Geometry check sheet. Reference: the model listing, model coordinates, mm. A direction names the side the tool comes from. Coordinates: 2 decimals unless noted, no trailing zeros. Order: outer loops, then holes, each group sorted by start corner. A loop starts at its lowest first (then second) coordinate and runs counter-clockwise, first axis right, second up. Notation, with made-up numbers: (-32.75, 3) - (10.25, 3) arc R23 cw to (10.25, 40) - close; hole circle Ø8 at (76.25, 23). An arc over 180 degrees is marked (long way). Put each result on its own line as item: value.
from build123d import *

# Parameters (mm, degrees)
SKETCH2_W           = 18.288
SKETCH2_H           = 40.64
BOSS_EXTRUDE1_DEPTH = 76.2
CUT_EXTRUDE1_REACH  = 90.275
SKETCH3_W           = 5.588
SKETCH3_H           = 6.35
SKETCH3_H_2         = 10.16
CUT_EXTRUDE2_REACH  = 89.289
SKETCH4_R           = 1.143
CUT_EXTRUDE3_REACH  = 90.275
SKETCH5_R           = 2.032
SKETCH6_R           = 5.08
CUT_EXTRUDE4_DEPTH  = 15.24
FILLET1_R           = 6.35
FILLET2_R           = 2.54
SKETCH7_R           = 3.81
CUT_EXTRUDE5_DEPTH  = 89.275141297


with BuildPart() as part:
    # Sketch2 → Boss-Extrude1 (new body)
    with BuildSketch(Plane(origin=(0, 0, 0), x_dir=(0, 0, -1), z_dir=(1, 0, 0))):
        with Locations((9.144, 20.32)):
            Rectangle(SKETCH2_W, SKETCH2_H)
    extrude(amount=BOSS_EXTRUDE1_DEPTH)

    # Sketch3 → Cut-Extrude1 (cut, up to next)
    with BuildSketch(Plane.ZY, mode=Mode.PRIVATE) as cut_extrude1_sk1:
        with Locations((-2.794, 37.465)):
            Rectangle(SKETCH3_W, SKETCH3_H)
    cut_extrude1_tool1 = extrude(cut_extrude1_sk1.sketch, amount=-CUT_EXTRUDE1_REACH, mode=Mode.PRIVATE) & part.part
    # Sketch3 → Cut-Extrude1 (cut, up to next)
    with BuildSketch(Plane.ZY, mode=Mode.PRIVATE) as cut_extrude1_sk2:
        with Locations((-2.794, 26.67)):
            Rectangle(SKETCH3_W, SKETCH3_H_2)
    cut_extrude1_tool2 = extrude(cut_extrude1_sk2.sketch, amount=-CUT_EXTRUDE1_REACH, mode=Mode.PRIVATE) & part.part
    add(cut_extrude1_tool1.solids().sort_by_distance((0, 37.465, -2.794))[0], mode=Mode.SUBTRACT)
    add(cut_extrude1_tool2.solids().sort_by_distance((0, 26.67, -2.794))[0], mode=Mode.SUBTRACT)

    # Sketch4 → Cut-Extrude2 (cut, up to next)
    with BuildSketch(Plane.XY.offset(-5.588), mode=Mode.PRIVATE) as cut_extrude2_sk1:
        with Locations((38.1, 24.13)):
            Circle(SKETCH4_R)
    cut_extrude2_tool1 = extrude(cut_extrude2_sk1.sketch, amount=-CUT_EXTRUDE2_REACH, mode=Mode.PRIVATE) & part.part
    add(cut_extrude2_tool1.solids().sort_by_distance((38.1, 24.13, -5.588))[0], mode=Mode.SUBTRACT)

    # Sketch5 → Cut-Extrude3 (cut, up to next)
    with BuildSketch(Plane(origin=(0, 40.64, 0), x_dir=(1, 0, 0), z_dir=(0, 1, 0)), mode=Mode.PRIVATE) as cut_extrude3_sk1:
        with Locations(Location((57.15, 11.938, 0), (0, 0, 270))):
            Circle(SKETCH5_R)
    cut_extrude3_tool1 = extrude(cut_extrude3_sk1.sketch, amount=-CUT_EXTRUDE3_REACH, mode=Mode.PRIVATE) & part.part
    # Sketch5 → Cut-Extrude3 (cut, up to next)
    with BuildSketch(Plane(origin=(0, 40.64, 0), x_dir=(1, 0, 0), z_dir=(0, 1, 0)), mode=Mode.PRIVATE) as cut_extrude3_sk2:
        with Locations(Location((19.05, 11.938, 0), (0, 0, 270))):
            Circle(SKETCH5_R)
    cut_extrude3_tool2 = extrude(cut_extrude3_sk2.sketch, amount=-CUT_EXTRUDE3_REACH, mode=Mode.PRIVATE) & part.part
    add(cut_extrude3_tool1.solids().sort_by_distance((57.15, 40.64, -11.938))[0], mode=Mode.SUBTRACT)
    add(cut_extrude3_tool2.solids().sort_by_distance((19.05, 40.64, -11.938))[0], mode=Mode.SUBTRACT)

    # Sketch6 → Cut-Extrude4 (cut)
    with BuildSketch(Plane(origin=(0, 40.64, 0), x_dir=(1, 0, 0), z_dir=(0, 1, 0))):
        with Locations(Location((19.05, 11.938, 0), (0, 0, 270))):
            Circle(SKETCH6_R)
        with Locations(Location((57.15, 11.938, 0), (0, 0, 270))):
            Circle(SKETCH6_R)
    extrude(amount=-CUT_EXTRUDE4_DEPTH, mode=Mode.SUBTRACT)

    # Fillet1
    # the kernel refuses this fillet: 6.35 mm, written as the material it takes off along each edge
    with BuildSketch(Plane(origin=(-15.875, 40.64, -18.288), x_dir=(0, -1, 0), z_dir=(1, 0, 0))) as fillet1_piece_1:
        with BuildLine():
            CenterArc((FILLET1_R, -FILLET1_R), FILLET1_R, 90, 90)
            Line((0, -FILLET1_R), (0, 0))
            Line((0, 0), (FILLET1_R, 0))
        make_face()
    extrude(amount=107.95, mode=Mode.SUBTRACT)

    # Fillet2
    fillet2_edges = [part.edges().sort_by_distance(p)[0] for p in [
        (38.1, 31.75, -5.588),
    ]]
    fillet(fillet2_edges, radius=FILLET2_R)

    # Sketch7 → Cut-Extrude5 (cut, through all)
    with BuildSketch(Plane.XZ):
        with Locations((2.54, -11.938)):
            Circle(SKETCH7_R)
        with Locations((73.66, -11.938)):
            Circle(SKETCH7_R)
    extrude(amount=-CUT_EXTRUDE5_DEPTH, mode=Mode.SUBTRACT)


solid = part.part
Q1. Depth check by flat-ended pin: pin 1 Ø2 at (x, z) = (17, -8) entering from -Y; pin 2 Ø2.5 at (x, y) = (20.5, 25) entering from +Z; pin 3 Ø6 at (x, z) = (2.54, -11.938) entering from +Y; pin 4 Ø8 at (x, z) = (19.05, -11.938) entering from +Y. Enter the tip coordinate at first touch or a pass-through.
Answer block:
pin 1: stops at y = 0
pin 2: stops at z = -5.59
pin 3: passes through
pin 4: stops at y = 25.4
Q2. Access from +Z, -Z, +X, -X, +Y, -Y to the whole of each face (thin tool, end or side, straight path). Record for faces 1 (the flat face through (38, 34.29, -3)), 2 (the cylindrical face through (38.63, 30.99, -4.86)), 3 (the flat face through (57.22, 25.4, -9.75)), 4 (the flat face through (38, 11, 0)).
Answer block:
face 1: +Z, +X, -X, +Y
face 2: +Z, +X, -X
face 3: +Y
face 4: +Z, +X, -X, +Y, -Y
Q3. Draft check along X on faces 5 (the flat face through (0, 20, -17)), 6 (the cylindrical face through (6.35, 20.04, -12.06)), 7 (the flat face through (38, 37, -5.588)). Enter one of: pulls with the +X half, pulls with the -X half, needs draft (parallel to the pull), parting line crosses it, or undercut.
Answer block:
face 5: pulls with the -X half
face 6: undercut
face 7: needs draft
Q4. Thickness scan on L1, parallel to Z at x = 19, y = 34; L2, parallel to X at y = 7, z = -11.25; L3, parallel to Y at x = 11, z = -2.75. Record the ranges inside material, lowest first. Write a range as [from, to].
Answer block:
L1: z = [-18.29, -17.02], [-6.86, 0]
L2: x = [6.29, 17.14], [20.96, 55.24], [59.06, 69.91]
L3: y = [0, 21.59], [31.75, 34.29]
Q5. Section check A-A on y = 24.13. Record the boundary of the cut face in (x, z).
Answer block:
outline: (0, -18.29) - (36.96, -18.29) - (36.96, -5.59) - (0, -5.59) - (0, -9.1) arc R3.81 cw (long way) to (0, -14.78) - close; (39.24, -18.29) - (76.2, -18.29) - (76.2, -14.78) arc R3.81 cw (long way) to (76.2, -9.1) - (76.2, -5.59) - (39.24, -5.59) - close; hole circle Ø4.06 at (19.05, -11.94); hole circle Ø4.06 at (57.15, -11.94)
Q6. Section check B-B on z = -12.75. Record the boundary of the cut face in (x, y), then the cut area to 3 significant figures.
Answer block:
outline: (6.26, 0) - (17.19, 0) - (17.19, 25.4) - (14.04, 25.4) - (14.04, 40.59) - (6.26, 40.59) - close; (20.91, 0) - (55.29, 0) - (55.29, 25.4) - (52.14, 25.4) - (52.14, 40.59) - (24.06, 40.59) - (24.06, 25.4) - (20.91, 25.4) - close; (59.01, 0) - (69.94, 0) - (69.94, 40.59) - (62.16, 40.59) - (62.16, 25.4) - (59.01, 25.4) - close; hole circle Ø2.29 at (38.1, 24.13)
area: 2,090 mm^2
Q7. Section check C-C on x = 19.05. Record the boundary of the cut face in (y, z).
Answer block:
outline: (0, -18.29) - (34.29, -18.29) arc R6.35 ccw to (38.1, -17.02) - (25.4, -17.02) - (25.4, -13.97) - (0, -13.97) - close; (0, -9.91) - (25.4, -9.91) - (25.4, -6.86) - (40.64, -6.86) - (40.64, -5.59) - (34.29, -5.59) - (34.29, 0) - (31.75, 0) - (31.75, -3.05) arc R2.54 cw to (29.21, -5.59) - (21.59, -5.59) - (21.59, 0) - (0, 0) - close
Q8. Section check D-D on y = 6.5. Record the boundary of the cut face in (x, z).
Answer block:
outline: (0, -18.29) - (76.2, -18.29) - (76.2, -14.78) arc R3.81 cw (long way) to (76.2, -9.1) - (76.2, 0) - (0, 0) - (0, -9.1) arc R3.81 cw (long way) to (0, -14.78) - close; hole circle Ø4.06 at (19.05, -11.94); hole circle Ø4.06 at (57.15, -11.94)
